from build123d import *

# Parameters (mm, degrees)
BOSS_EXTRUDE1_DEPTH     = 370
SKETCH9_W               = 58
SKETCH9_H               = 50
SKETCH9_H_2             = 51
BOSS_EXTRUDE2_DEPTH     = 4
SKETCH14_R              = 5
BOSS_EXTRUDE3_DEPTH     = 49
CUT_EXTRUDE4_REACH      = 377.391
SKETCH15_W              = 25
SKETCH15_H              = 30
SKETCH15_W_2            = 30
SKETCH15_H_2            = 67.188472817
SKETCH16_R              = 4
CUT_EXTRUDE5_DEPTH      = 376.049663378
CUT_EXTRUDE6_DEPTH      = 376.049663378
CUT_EXTRUDE7_DEPTH      = 375.841633227
CUT_EXTRUDE7_DEPTH_BACK = 375.841633227
SKETCH18_R              = 5
CUT_EXTRUDE8_DEPTH      = 12.5


with BuildPart() as part:
    # Sketch3 → Boss-Extrude1 (new body)
    with BuildSketch(Plane(origin=(0, 0, 0), x_dir=(1, 0, 0), z_dir=(0, 1, 0))):
        Polygon((0, 0), (-49, 0), (-49, 34), (-45, 34), (-45, 4), (-4, 4), (-4, 34), (0, 34), align=None)
    extrude(amount=BOSS_EXTRUDE1_DEPTH)

    # Sketch9 → Boss-Extrude2 (add)
    with BuildSketch(Plane.XY):
        with Locations((-24.5, 345)):
            Rectangle(SKETCH9_W, SKETCH9_H)
        with Locations((-24.5, 38.5)):
            Rectangle(SKETCH9_W, SKETCH9_H_2)
    extrude(amount=-BOSS_EXTRUDE2_DEPTH)

    # Sketch14 → Boss-Extrude3 (add)
    # profile 1 of 2: a face of its own
    with BuildSketch(Plane(origin=(0, 0, 0), x_dir=(0, 0, -1), z_dir=(1, 0, 0))):
        with BuildLine():
            Line((19, 360.05579248), (19, 344.94420752))
            ThreePointArc((19, 344.94420752), (12, 342.2), (5, 344.94420752))
            Line((5, 344.94420752), (5, 360.05579248))
            ThreePointArc((5, 360.05579248), (12, 362.8), (19, 360.05579248))
        make_face()
        with Locations((12, 352.5)):
            Circle(SKETCH14_R, mode=Mode.SUBTRACT)
    # profile 2 of 2: a face of its own
    with BuildSketch(Plane(origin=(0, 0, 0), x_dir=(0, 0, -1), z_dir=(1, 0, 0))):
        with BuildLine():
            Line((29.5, 38.5), (29.5, 27.627016654))
            ThreePointArc((29.5, 27.627016654), (15.608560863, 27.436987987), (22.5, 39.5))
            Line((22.5, 39.5), (28.5, 39.5))
            Line((28.5, 39.5), (29.5, 38.5))
        make_face()
        with BuildLine():
            Line((27.5, 34.81662479), (27.5, 28.18337521))
            ThreePointArc((27.5, 28.18337521), (22.5, 25.5), (17.5, 28.18337521))
            Line((17.5, 28.18337521), (17.5, 34.81662479))
            ThreePointArc((17.5, 34.81662479), (22.5, 37.5), (27.5, 34.81662479))
        make_face(mode=Mode.SUBTRACT)
    extrude(amount=-BOSS_EXTRUDE3_DEPTH)

    # Cut-Extrude4: up to this face of the body (flat: up to its plane)
    cut_extrude4_end = Plane(part.part.faces().sort_by_distance((-24.5, 185, -4))[0])
    # Sketch15 → Cut-Extrude4 (cut, up to the picked face)
    with BuildSketch(Plane(origin=(0, 0, -34), x_dir=(-1, 0, 0), z_dir=(0, 0, -1)), mode=Mode.PRIVATE) as cut_extrude4_sk1:
        with Locations((24.5, 355)):
            Rectangle(SKETCH15_W, SKETCH15_H)
    cut_extrude4_tool1 = split(extrude(cut_extrude4_sk1.sketch, amount=-CUT_EXTRUDE4_REACH, mode=Mode.PRIVATE), bisect_by=cut_extrude4_end, keep=Keep.BOTH, mode=Mode.PRIVATE)
    # Sketch15 → Cut-Extrude4 (cut, up to the picked face)
    with BuildSketch(Plane(origin=(0, 0, -34), x_dir=(-1, 0, 0), z_dir=(0, 0, -1)), mode=Mode.PRIVATE) as cut_extrude4_sk2:
        with Locations((24.5, 33.594236409)):
            Rectangle(SKETCH15_W_2, SKETCH15_H_2)
    cut_extrude4_tool2 = split(extrude(cut_extrude4_sk2.sketch, amount=-CUT_EXTRUDE4_REACH, mode=Mode.PRIVATE), bisect_by=cut_extrude4_end, keep=Keep.BOTH, mode=Mode.PRIVATE)
    add(cut_extrude4_tool1.solids().sort_by(Axis((-24.5, 355, -34), (0, 0, 1)))[0], mode=Mode.SUBTRACT)
    add(cut_extrude4_tool2.solids().sort_by(Axis((-24.5, 33.594236, -34), (0, 0, 1)))[0], mode=Mode.SUBTRACT)

    # Sketch16 → Cut-Extrude5 (cut, through all)
    with BuildSketch(Plane(origin=(0, 0, -4), x_dir=(-1, 0, 0), z_dir=(0, 0, -1))):
        with Locations((24.5, 85)):
            Circle(SKETCH16_R)
        with Locations((24.5, 308)):
            Circle(SKETCH16_R)
    extrude(amount=-CUT_EXTRUDE5_DEPTH, mode=Mode.SUBTRACT)

    # Sketch17 → Cut-Extrude6 (cut, through all)
    with BuildSketch(Plane(origin=(0, 0, -4), x_dir=(-1, 0, 0), z_dir=(0, 0, -1))):
        with BuildLine():
            Line((19.5, 236.590169944), (19.5, 225.409830056))
            ThreePointArc((19.5, 225.409830056), (24.5, 223.5), (29.5, 225.409830056))
            Line((29.5, 225.409830056), (29.5, 236.590169944))
            ThreePointArc((29.5, 236.590169944), (24.5, 238.5), (19.5, 236.590169944))
        make_face()
    extrude(amount=-CUT_EXTRUDE6_DEPTH, mode=Mode.SUBTRACT)

    # Sketch18 → Cut-Extrude7 (cut, two sides: drawn at the far end of the back side and taken through both)
    with BuildSketch(Plane(origin=(-45, 0, 0), x_dir=(0, 0, -1), z_dir=(1, 0, 0)).offset(-CUT_EXTRUDE7_DEPTH_BACK)):
        with Locations(Location((12, 352.5, 0), (0, 0, 90))):
            Circle(SKETCH18_R)
        with BuildLine():
            Line((17.5, 34.81662479), (17.5, 28.18337521))
            ThreePointArc((17.5, 28.18337521), (22.5, 25.5), (27.5, 28.18337521))
            Line((27.5, 28.18337521), (27.5, 34.81662479))
            ThreePointArc((27.5, 34.81662479), (22.5, 37.5), (17.5, 34.81662479))
        make_face()
    extrude(amount=CUT_EXTRUDE7_DEPTH + CUT_EXTRUDE7_DEPTH_BACK, mode=Mode.SUBTRACT)

    # Sketch19 → Cut-Extrude8 (cut, symmetric)
    with BuildSketch(Plane(origin=(-24.5, 0, 0), x_dir=(0, 0, -1), z_dir=(1, 0, 0))):
        with BuildLine():
            Line((4, 370), (4, 338.5))
            ThreePointArc((4, 338.5), (2.502016162, 346.278692991), (2, 354.184387141))
            Line((2, 354.184387141), (2, 370))
            Line((2, 370), (4, 370))
        make_face()
    extrude(amount=CUT_EXTRUDE8_DEPTH, both=True, mode=Mode.SUBTRACT)


solid = part.part
Geometry check sheet. Reference: the model listing, model coordinates, mm. A direction names the side the tool comes from. Round coordinates to 2 decimals unless told otherwise and drop trailing zeros. Order: outer loops, then holes, each group sorted by start corner. A loop starts at its lowest first (then second) coordinate and runs counter-clockwise, first axis right, second up. Notation, with made-up numbers: M 14.25,10.25 L 48.25,10.25 A24 cw 48.25,30.25 Z; hole C 74.25,19.5 d7. An arc over 180 degrees is marked long. Write each question's results on one line, items separated by ' | '. Start each with the question number.
1. Material ranges on L1, parallel to Y at x = -24, z = -1; L2, parallel to X at y = 308, z = -3; L3, parallel to X at y = 163, z = -32, recorded low to high. Write a range as from..to.
2. Cross-section at C-C on y = 242.5. Record the boundary of the cut face in (x, z).
3. Draft check along Y on faces 5 (the face through (-44, 31, -27.5)), 6 (the face through (-25, 182, -4)), 7 (the face through (-7.9, 362.8, -11.9)). Enter one of: pulls with the +Y half, pulls with the -Y half, needs draft (parallel to the pull), parting line crosses it, or undercut.
4. Cross-section at A-A on y = 85. Record the boundary of the cut face in (x, z).
5. Cross-section at B-B on x = -24.5. Record the boundary of the cut face in (y, z).
6. Set-up check for faces 1 (the face through (-41, 352, -5)), 2 (the face through (-44.3, 37.5, -22.6)), 3 (the face through (-7.9, 342.2, -12.1)), 4 (the face through (-24.325, 346.169, -2.516)): record each of +Z, -Z, +X, -X, +Y, -Y from which the full face is reachable in a straight line by a thin tool's end or side.
7. Go/stop test with flat-tipped pins: P1, Ø4.5, axis at y = 230, z = -3, coming from the +X side; P2, Ø2, axis at y = 158, z = -27.5, coming from the -X side; P3, Ø10, axis at y = 55, z = -5, coming from the +X side; P4, Ø2, axis at x = -26, y = 77, coming from the -Z side. Record where each tip stops, or that it passes through.
Resolved:
1) L1: 0..81.03, 88.97..223.52, 238.48..304.03, 311.97..370 | L2: -49..-28.5, -20.5..0 | L3: -49..-45, -4..0
2) outline: M -49,-34 L -45,-34 L -45,-4 L -4,-4 L -4,-34 L 0,-34 L 0,0 L -49,0 Z
3) face 5: undercut | face 6: needs draft | face 7: pulls with the +Y half
4) outline: M -49,-34 L -45,-34 L -45,-4 L -28.5,-4 L -28.5,0 L -49,0 Z; M -20.5,-4 L -4,-4 L -4,-34 L 0,-34 L 0,0 L -20.5,0 Z
5) outline: M 0,-4 L 81,-4 L 81,0 L 0,0 Z; M 89,-4 L 223.5,-4 L 223.5,0 L 89,0 Z; M 238.5,-4 L 304,-4 L 304,0 L 238.5,0 Z; M 312,-4 L 338.5,-4 A62.5 cw 354.18,-2 L 370,-2 L 370,0 L 312,0 Z
6) face 1: +Y, -Y | face 2: +X, -X | face 3: none | face 4: -Z, +Y
7) P1: x = 0 | P2: x = -49 | P3: x = 4.5 | P4: z = -4
